from build123d import *

# Parameters (mm, degrees)
F0_W = 23
F0_H = 6.5


with BuildPart() as f1:
    # F0 (on Top) → F1 (revolve)
    with BuildSketch(Plane.XY):
        with BuildLine():
            Line((-61, 0), (-61, -6.5))
            Line((-61, -6.5), (-61, -10))
            Line((-61, -10), (-48, -10))
            ThreePointArc((-48, -10), (-35.155125, -8.767246), (-22.638298, -11.904051))
            ThreePointArc((-22.638298, -11.904051), (6.129777, -16.34737), (33.24159, -5.750445))
            ThreePointArc((33.24159, -5.750445), (35.378368, -3.221045), (36.145537, 0))
            Line((36.145537, 0), (-61, 0))
        make_face()
    revolve(axis=Axis((-4.224361, 0, 0), (1, 0, 0)))

    # F0 (on Top) → F2 (revolve)
    with BuildSketch(Plane.XY):
        with Locations((-72.5, -3.25)):
            Rectangle(F0_W, F0_H)
    revolve(axis=Axis((-4.224361, 0, 0), (1, 0, 0)))


solid = f1.part
Geometry check sheet. Reference: the model listing, model coordinates, mm. A direction names the side the tool comes from. Give positions to 0.01 mm unless a question says otherwise; leave off trailing zeros. Order: outer loops, then holes, each group sorted by start corner. A loop starts at its lowest first (then second) coordinate and runs counter-clockwise, first axis right, second up. Notation, with made-up numbers: (18.25, 59.25) - (50.25, 59.25) arc R14 cw to (50.25, 68.25) - close; hole circle Ø11 at (81, 7). An arc over 180 degrees is marked (long way). Answer as a JSON object with one key per item and string values.
(1) Cross-section at A-A (x = -58). Record the cut outline in (y, z), then the cut area to 3 significant figures.
Report:
{"outline": "circle Ø20 at (0, 0)", "area": "314 mm^2"}
(2) Depth check by flat-ended pin: pin 1 Ø5 at (x, z) = (-65, 5.5) entering from +Y; pin 2 Ø8 at (x, y) = (16, 3) entering from +Z; pin 3 Ø8 at (y, z) = (13, -7.5) entering from +X. Enter the tip coordinate at first touch or a pass-through.
Report:
{"pin 1": "y = 5.77", "pin 2": "z = 15.24", "pin 3": "x = 24.57"}
(3) Cross-section at B-B (x = -27). Record the cut outline in (y, z).
Report:
{"outline": "circle Ø20.58 at (0, 0)"}
(4) Material ranges on line 1 (Z direction, x = -67, y = 3); line 2 (Y direction, x = -77, z = -0.5); line 3 (X direction, y = -4.5, z = -6.5), recorded low to high.
Report:
{"line 1": "-5.77 to 5.77", "line 2": "-6.48 to 6.48", "line 3": "-61 to 30.1"}
(5) Tool access check on faces 1 (the flat face through (-84, 0, 0)), 2 (the cylindrical face through (-72.339, 5.158, 3.955)). Record the directions out of +Z, -Z, +X, -X, +Y, -Y that give a thin tool (end or side, any length) a straight path to the whole face; none if there is none.
Report:
{"face 1": "+Z, -Z, -X, +Y, -Y", "face 2": "-X"}
(6) Draft check along Y on faces 3 (the cylindrical face through (-54.41, 2.17, 9.76)), 4 (the flat face through (-61, 7, 0)). Enter one of: released by +Y, released by -Y, zero draft, split by the parting line, or undercut.
Report:
{"face 3": "split by the parting line", "face 4": "zero draft"}
